Could you check a few things on this model? Use its own coordinates, in mm. A direction names the side the tool comes from. Give positions to 0.01 mm unless a question says otherwise; leave off trailing zeros. Write each loop counter-clockwise with the first axis right and the second up, starting at its lowest first coordinate (ties: lowest second). Pieces come first, ordered by that corner, then holes. Notation, with made-up numbers: M -26,-1 L -1,-1 A20 ccw -1,22 Z; hole C -36.5,24 d8. An arc over 180 degrees is marked long. Use one line per item in the form item = value.
from build123d import *

# Parameters (mm, degrees)
PAD_DEPTH            = 25
SKETCH001_R          = 1.9
POCKET_DEPTH         = 25
SKETCH002_W          = 20
SKETCH002_H          = 20
POCKET001_DEPTH      = 20
SKETCH003_W          = 19.75
SKETCH003_H          = 11.5
SKETCH003_W_2        = 11.5
SKETCH003_H_2        = 19.75
POCKET002_DEPTH      = 20
BODY_PLACEMENT_ANGLE = 90


with BuildPart() as part:
    # Sketch → Pad (new body)
    with BuildSketch(Plane.XY):
        Polygon((0, 23.75), (23.75, 23.75), (23.75, 0), (43.75, 0), (43.75, 43.75), (0, 43.75), align=None)
    extrude(amount=PAD_DEPTH)

    # Sketch001 (on Face8 of Pad) → Pocket (cut)
    with BuildSketch(Plane.XY.offset(25)):
        with Locations((33.75, 33.75)):
            Circle(SKETCH001_R)
    extrude(amount=-POCKET_DEPTH, mode=Mode.SUBTRACT)

    # Sketch002 (on Face5 of Pocket) → Pocket001 (cut)
    with BuildSketch(Plane.XY.offset(25)):
        with Locations((38.25, 38.25)):
            Rectangle(SKETCH002_W, SKETCH002_H)
    extrude(amount=-POCKET001_DEPTH, mode=Mode.SUBTRACT)

    # Sketch003 (on Face5 of Pocket001) → Pocket002 (cut)
    with BuildSketch(Plane.XY.offset(25)):
        with Locations((14.125, 33.75)):
            Rectangle(SKETCH003_W, SKETCH003_H)
        with Locations((33.75, 14.125)):
            Rectangle(SKETCH003_W_2, SKETCH003_H_2)
    extrude(amount=-POCKET002_DEPTH, mode=Mode.SUBTRACT)


with BuildPart() as part_1:
    # Body placement: moved
    add(part.part.rotate(Axis((0, 0, 0), (0, 0, -1)), BODY_PLACEMENT_ANGLE))


solid = part_1.part
1) I want a section at B-B, the plane y = -33.75. Please give me the cut outline in (x, z), plus the area to 3 significant figures.
Checked values:
outline = M 0,0 L 31.85,0 L 31.85,5 L 28.25,5 L 28.25,25 L 24,25 L 24,5 L 4.25,5 L 4.25,25 L 0,25 Z; M 35.65,0 L 43.75,0 L 43.75,5 L 35.65,5 Z
area = 370 mm2
2) For pin 1 Ø4.5 at (x, y) = (33.75, -33.75) entering from -Z; pin 2 Ø2 at (y, z) = (-32, 12) entering from +X; pin 3 Ø10 at (y, z) = (-14.5, 10.5) entering from -X; pin 4 Ø12 at (x, z) = (14.5, 6.5) entering from +Y, each with a flat end and sliding along its axis, tell me the tip position at first contact or that it passes through.
Checked values:
pin_1 = 0
pin_2 = 28.25
pin_3 = 23.75
pin_4 = -23.75
3) Thinking about a two-plate mould opening in X: for faces 1 (the flat face through (0, -34, 12)), 2 (the flat face through (4.25, -34, 15)), 3 (the flat face through (36, -36, 5)), which applies, released by +X, released by -X, zero draft, split by the parting line, or undercut?
Checked values:
face_1 = released by -X
face_2 = undercut
face_3 = zero draft
4) If I drill on L1, parallel to X at y = -33.75, z = 1.65; L2, parallel to Y at x = 10.5, z = 5.75, over which ranges is the centre line in solid material (lowest first)?
Checked values:
L1 = 0 to 31.85, 35.65 to 43.75
L2 = -43.75 to -39.5, -28 to -23.75
5) For faces 4 (the flat face through (23.75, -12, 12)), 5 (the flat face through (14, -39.5, 15)), 6 (the flat face through (22, -26, 25)), 7 (the flat face through (28.25, -36, 15)), which set-ups out of +Z, -Z, +X, -X, +Y, -Y let a thin tool reach every point of the face, with its end or its side?
Checked values:
face_4 = +Z, -Z, -X, +Y
face_5 = +Z
face_6 = +Z, +X, -X, +Y, -Y
face_7 = +Z, +X, -Y
6) I want a section at D-D, the plane y = -14.5. Please give me the cut outline in (x, z).
Checked values:
outline = M 23.75,0 L 43.75,0 L 43.75,25 L 39.5,25 L 39.5,5 L 28,5 L 28,25 L 23.75,25 Z
7) I want a section at A-A, the plane x = 33.75. Please give me the cut outline in (y, z), plus the area to 3 significant figures.
Checked values:
outline = M -43.75,0 L -35.65,0 L -35.65,5 L -43.75,5 Z; M -31.85,0 L 0,0 L 0,25 L -4.25,25 L -4.25,5 L -24,5 L -24,25 L -28.25,25 L -28.25,5 L -31.85,5 Z
area = 370 mm2
8) I want a section at C-C, the plane z = 19.5. Please give me the cut outline in (x, y).
Checked values:
outline = M 0,-43.75 L 28.25,-43.75 L 28.25,-28.25 L 43.75,-28.25 L 43.75,0 L 23.75,0 L 23.75,-23.75 L 0,-23.75 Z; hole M 4.25,-39.5 L 24,-39.5 L 24,-28 L 4.25,-28 Z; hole M 28,-24 L 39.5,-24 L 39.5,-4.25 L 28,-4.25 Z
